Work out the finished part from the listing and answer in its coordinate system (mm). Face numbers are marked on the shaded views. A direction names the side the tool comes from. Round coordinates to 2 decimals unless told otherwise and drop trailing zeros. Loops run counter-clockwise (first coordinate to the right, second up) from the corner with the lowest first, then second, coordinate; pieces in that order, holes last. Notation, with made-up numbers: (21.25, 43.25) - (62.25, 43.25) arc R15 ccw to (62.25, 51.25) - close; hole circle Ø10 at (45, 41.25). An arc over 180 degrees is marked (long way). Return JSON: item names as keys, results as strings.
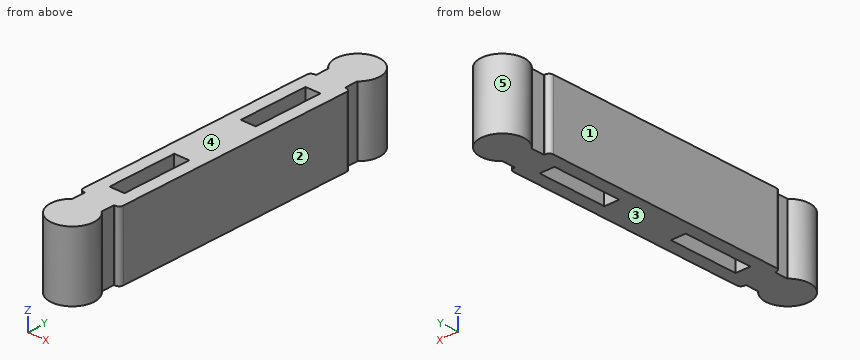
from build123d import *

# Parameters (mm, degrees)
F0_R     = 3.302
F1_DEPTH = 10.16
F3_DEPTH = 10.16
F4_W     = 6.096
F4_H     = 19.05
F5_DEPTH = 10.16
F6_R     = 0.635
F7_W     = 2.286
F7_H     = 10.668
F8_DEPTH = 25.4


with BuildPart() as f1:
    # F0 (on Top) → F1 (new body)
    with BuildSketch(Plane.XY):
        Circle(F0_R)
    extrude(amount=F1_DEPTH)

    # F2 (on face) → F3 (join, through all)
    with BuildSketch(Plane(origin=(0, 0, 0), x_dir=(1, 0, 0), z_dir=(0, 0, -1))):
        with BuildLine():
            ThreePointArc((2.2225, -2.442068), (0, -3.302), (-2.2225, -2.442068))
            Line((-2.2225, -2.442068), (-2.2225, -4.474068))
            Line((-2.2225, -4.474068), (2.2225, -4.474068))
            Line((2.2225, -4.474068), (2.2225, -2.442068))
        make_face()
    extrude(amount=-F3_DEPTH)

    # F4 (on Top) → F5 (join, through all)
    with BuildSketch(Plane.XY):
        with Locations((0, 13.999068)):
            Rectangle(F4_W, F4_H)
    extrude(amount=F5_DEPTH)

    # F6
    f6_edges = [f1.edges().sort_by_distance(p)[0] for p in [
        (3.048, 4.474068, 5.08),
        (-3.048, 4.474068, 5.08),
    ]]
    fillet(f6_edges, radius=F6_R)

    # F7 (on face) → F8 (cut)
    with BuildSketch(Plane.XY.offset(10.16)):
        with Locations((0, 12.7)):
            Rectangle(F7_W, F7_H)
    extrude(amount=-F8_DEPTH, mode=Mode.SUBTRACT)

    # F9: F1 across face


with BuildPart() as f1_1:
    add(f1.part)
    add(f1.part.mirror(Plane(origin=(0, 23.524068, 5.08), x_dir=(-1, 0, 0), z_dir=(0, 1, 0))))


solid = f1_1.part
1) Find the intervals of material crossed by L1, parallel to Y at x = 0.25, z = 5.75; L2, parallel to X at y = 8.5, z = 9; L3, parallel to Y at x = 2.75, z = 1.5, in increasing order.
Verdict:
{"L1": "y = -3.29 to 7.37, 18.03 to 29.01, 39.68 to 50.34", "L2": "x = -3.05 to -1.14, 1.14 to 3.05", "L3": "y = -1.83 to 1.83, 4.57 to 42.48, 45.22 to 48.88"}
2) A tool of negligible diameter and unlimited length cuts with its end or side. For the marked faces 1, 2 and 3, from which of +Z, -Z, +X, -X, +Y, -Y can it reach the whole face along a straight path? Write none if from no direction.
Verdict:
{"face 1": "+Z, -Z, -X", "face 2": "+Z, -Z, +X", "face 3": "-Z, +X, -X, +Y, -Y"}
3) Section A-A (x = 0) is taken. Give the vertices of the cut face in (y, z).
Verdict:
{"outline": "(-3.3, 0) - (7.37, 0) - (7.37, 10.16) - (-3.3, 10.16) - close; (18.03, 0) - (29.01, 0) - (29.01, 10.16) - (18.03, 10.16) - close; (39.68, 0) - (50.35, 0) - (50.35, 10.16) - (39.68, 10.16) - close"}
4) Determine the mould class of the marked faces 4 and 5 for opening direction Y: pulls with the +Y half, pulls with the -Y half, needs draft (parallel to the pull), parting line crosses it, or undercut.
Verdict:
{"face 4": "needs draft", "face 5": "undercut"}
5) Section B-B (y = 35) is taken. Give the vertices of the cut face in (x, z), and give its area (3 significant figures).
Verdict:
{"outline": "(-3.05, 0) - (-1.14, 0) - (-1.14, 10.16) - (-3.05, 10.16) - close; (1.14, 0) - (3.05, 0) - (3.05, 10.16) - (1.14, 10.16) - close", "area": "38.7 mm2"}
6) Flat-ended cylindrical pins translate along their axes: pin 1 (0.7 mm diameter, centred on x = -0.5, z = 3.5, fed in from -Y); pin 2 (3 mm diameter, centred on y = 3.5, z = 5, fed in from -X); pin 3 (1 mm diameter, centred on y = 3.5, z = 7, fed in from +X). Find the tip coordinate at first contact, or state that the pin passes through.
Verdict:
{"pin 1": "stops at y = -3.3", "pin 2": "stops at x = -3.04", "pin 3": "stops at x = 2.22"}
7) Section D-D (y = 45.5) is taken. Give the vertices of the cut face in (x, z).
Verdict:
{"outline": "(-2.92, 0) - (2.92, 0) - (2.92, 10.16) - (-2.92, 10.16) - close"}
8) Section C-C (z = 1) is taken. Count the separate pieces of the cut face and the enclosed holes in it, and give its area (3 significant figures).
Verdict:
{"separate pieces": "1", "enclosed holes": "2", "area": "264 mm2"}
